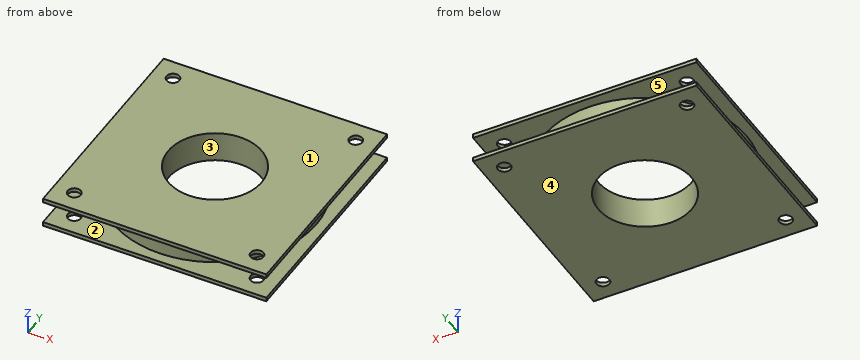
Solid Edge part; units mm, degrees
sketch "Sketch1" plane through (0, 0, 0) normal (0, 0, 1) x (1, 0, 0)
  line L0 (27.5, -27.5) -> (-27.5, -27.5)
  line L1 (-27.5, -27.5) -> (-27.5, 27.5)
  line L2 (-27.5, 27.5) -> (27.5, 27.5)
  line L3 (27.5, 27.5) -> (27.5, -27.5)
  dimension "D1" = 27.5
  dimension "D2" = 27.5
extrude "Protrusion1" add sketch "Sketch1" along normal blind 7.5
sketch "Sketch2" plane through (0, 0, 6.5) normal (0, 0, 1) x (1, 0, 0)
  circle A0 centre (0, 0) radius 25
extrude "ExtrudedCutout_1" cut sketch "Sketch2" against normal blind 5.5 flip side to cut
hole "Hole_1" at (0, 0, 7.5) direction (0, 0, -1) diameter 23 end through all
hole "Hole_2" at (-22.5, 22.5, 7.5) direction (0, 0, -1) diameter 3.2 end through all
hole "Hole1" at (-22.5, -22.5, 7.5) direction (0, 0, -1) diameter 3.2 end through all
hole "Hole2" at (22.5, -22.5, 7.5) direction (0, 0, -1) diameter 3.2 end through all
hole "Hole3" at (22.5, 22.5, 7.5) direction (0, 0, -1) diameter 3.2 end through all
Source: CAD feature listing. Evaluate the final solid. Frame: model axes, mm. Face numbers are marked on the shaded views. A direction names the side the tool comes from. Round coordinates to 2 decimals unless told otherwise and drop trailing zeros. Loops run counter-clockwise (first coordinate to the right, second up) from the corner with the lowest first, then second, coordinate; pieces in that order, holes last. Notation, with made-up numbers: M -25,58.5 L 10,58.5 A5 cw 10,62.5 Z; hole C 0,-4.5 d6. An arc over 180 degrees is marked long. Return JSON: item names as keys, results as strings. Group by question number.
1. Mould query, pull axis Z, two halves, no side actions, for the marked faces 1, 2 and 3. Classes: released by +Z, released by -Z, zero draft, split by the parting line, or undercut.
2. Material intervals for line 1 along X through (y, z) = (-22.5, 0.8); line 2 along Z through (x, y) = (25, -13), sorted ascending. Write a range as from..to.
3. Pin query (flat end, axial travel): pin 1 (1.5 mm diameter, centred on x = -10, z = 4.5, fed in from -Y); pin 2 (1 mm diameter, centred on x = 19.5, z = 4, fed in from +Y). Return the tip coordinate at first contact, or that it passes through.
4. Section query A-A on x = -22.5. Output: boundary loops of the cut face in (y, z), and give its area (3 significant figures).
5. Reachability of the marked faces 4 and 5 from +Z, -Z, +X, -X, +Y, -Y: full face, straight path, thin tool, end or side. Return the list, or none.
6. Section query C-C on x = 0. Output: boundary loops of the cut face in (y, z), and give its area (4 significant figures).
Checks:
{
 "1": {"face 1": "released by +Z", "face 2": "undercut", "face 3": "zero draft"},
 "2": {"line 1": "x = -27.5..-24.1, -20.9..20.9, 24.1..27.5", "line 2": "z = 0..1, 6.5..7.5"},
 "3": {"pin 1": "stops at y = -23.23", "pin 2": "stops at y = 16.25"},
 "4": {"outline": "M -27.5,0 L -24.1,0 L -24.1,1 L -27.5,1 Z; M -27.5,6.5 L -24.1,6.5 L -24.1,7.5 L -27.5,7.5 Z; M -20.9,0 L 20.9,0 L 20.9,1 L 10.9,1 L 10.9,6.5 L 20.9,6.5 L 20.9,7.5 L -20.9,7.5 L -20.9,6.5 L -10.9,6.5 L -10.9,1 L -20.9,1 Z; M 24.1,0 L 27.5,0 L 27.5,1 L 24.1,1 Z; M 24.1,6.5 L 27.5,6.5 L 27.5,7.5 L 24.1,7.5 Z", "area": "217 mm²"},
 "5": {"face 4": "-Z, +X, -X, +Y, -Y", "face 5": "none"},
 "6": {"outline": "M -27.5,0 L -11.5,0 L -11.5,7.5 L -27.5,7.5 L -27.5,6.5 L -25,6.5 L -25,1 L -27.5,1 Z; M 11.5,0 L 27.5,0 L 27.5,1 L 25,1 L 25,6.5 L 27.5,6.5 L 27.5,7.5 L 11.5,7.5 Z", "area": "212.5 mm²"}
}
